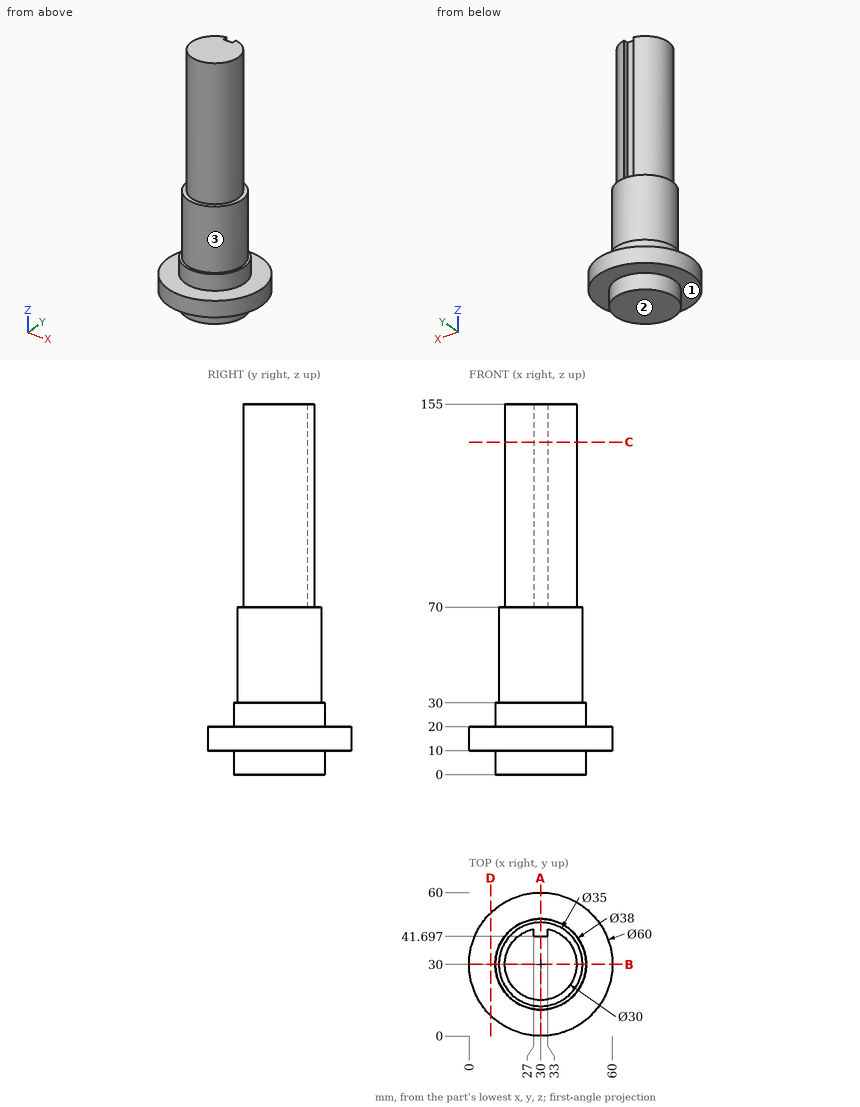
Study the drawing (mm; zero at the part's minimum x, y, z) and answer. A direction names the side the tool comes from. Coordinates: 2 decimals unless noted, no trailing zeros. Order: outer loops, then holes, each group sorted by start corner. A loop starts at its lowest first (then second) coordinate and runs counter-clockwise, first axis right, second up. Notation, with made-up numbers: (33.25, 21) -> (37.25, 21) arc R25 ccw to (37.25, 45) -> close; hole circle Ø1 at (23.5, 51). An arc over 180 degrees is marked (long way). Answer in a Markdown table with one row per item. Add a question column.
Item 1: Find section B-B (y = 30). Write down the section's boundary in (x, z), then the cut area to 3 significant figures.
Item 2: Which of the six approach directions +Z, -Z, +X, -X, +Y, -Y give full straight-line access (tool end or side, diameter ignored) to the marked faces 1, 2 and 3?
Item 3: Each of these flat-tipped pins is pushed along its axis until it touches: P1, Ø6, axis at x = 26.5, z = 99, coming from the -Y side; P2, Ø1.8, axis at x = 29, z = 99.5, coming from the +Y side; P3, Ø3.5, axis at y = 43.5, z = 98, coming from the +X side. Where does it stop, or does it pass through?
Item 4: Find the intervals of material crossed by L1, parallel to Z at x = 12.5, y = 49; L2, parallel to Z at x = 20, y = 16.5; L3, parallel to Y at x = 41, z = 16, in increasing order. Write a range as from..to.
Item 5: Find section D-D (x = 9). Write down the section's boundary in (y, z).
Item 6: Find section A-A (x = 30). Write down the section's boundary in (y, z).
Item 7: Find section C-C (z = 139). Write down the section's boundary in (x, y).
Result set:
| question | item | result |
|---|---|---|
| 1 | outline | (0, 10) -> (11, 10) -> (11, 0) -> (49, 0) -> (49, 10) -> (60, 10) -> (60, 20) -> (49, 20) -> (49, 30) -> (47.5, 30) -> (47.5, 70) -> (45, 70) -> (45, 155) -> (15, 155) -> (15, 70) -> (12.5, 70) -> (12.5, 30) -> (11, 30) -> (11, 20) -> (0, 20) -> close |
| 1 | area | 5,310 mm² |
| 2 | face 1 | -Z |
| 2 | face 2 | -Z, +X, -X, +Y, -Y |
| 2 | face 3 | +Z |
| 3 | P1 | stops at y = 15.01 |
| 3 | P2 | stops at y = 41.7 |
| 3 | P3 | stops at x = 39.32 |
| 4 | L1 | z = 10..20 |
| 4 | L2 | z = 0..70 |
| 4 | L3 | y = 2.09..57.91 |
| 5 | outline | (8.58, 10) -> (51.42, 10) -> (51.42, 20) -> (8.58, 20) -> close |
| 6 | outline | (0, 10) -> (11, 10) -> (11, 0) -> (49, 0) -> (49, 10) -> (60, 10) -> (60, 20) -> (49, 20) -> (49, 30) -> (47.5, 30) -> (47.5, 70) -> (41.7, 70) -> (41.7, 155) -> (15, 155) -> (15, 70) -> (12.5, 70) -> (12.5, 30) -> (11, 30) -> (11, 20) -> (0, 20) -> close |
| 7 | outline | (27, 41.7) -> (27, 44.7) arc R15 ccw (long way) to (33, 44.7) -> (33, 41.7) -> close |
